For this review, take the finished solid that the model builds, in its own axes (mm). Give positions to 0.01 mm unless a question says otherwise; leave off trailing zeros. Loops run counter-clockwise (first coordinate to the right, second up) from the corner with the lowest first, then second, coordinate; pieces in that order, holes last. Notation, with made-up numbers: (35, 71) - (48, 71) arc R5 ccw to (48, 79) - close; hole circle Ø4 at (14.5, 80.5). An arc over 180 degrees is marked (long way). Answer in a Markdown table with one row per item.
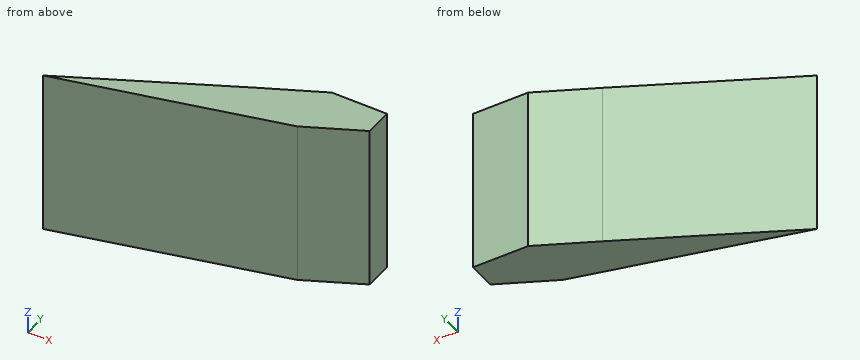
Autodesk Fusion 360 part; units mm, degrees
sketch "Sketch4" plane through (0, 0, 0) normal (0, 0, 1) x (1, 0, 0)
  line L0 (0, 0) -> (30, 0)
  line L1 (30, 0) -> (30, 10)
  line L2 (30, 10) -> (0, 10)
  line L3 (0, 10) -> (0, 0)
sketch "Sketch5" plane through (0, 0, 0) normal (0, 0, 1) x (1, 0, 0)
  line L0 (0, 0) -> (20, 5)
  line L1 (20, 5) -> (25.0128, 7.4566)
  line L2 (25.0128, 7.4566) -> (25.0128, 10)
  line L3 (25.0128, 10) -> (20, 10)
  line L4 (20, 10) -> (14.8103, 7.4566)
  line L5 (14.8103, 7.4566) -> (0, 0)
extrude "Extrude9" add sketch "Sketch5" along normal blind 15
1. We need section C-C, the plane y = 4. Give the boundary of the cut face in (x, z), and give its area (3 significant figures).
Values:
| item | result |
|---|---|
| outline | (7.94, 0) - (16, 0) - (16, 15) - (7.94, 15) - close |
| area | 121 mm^2 |
2. We need section B-B, the plane x = 2. Give the boundary of the cut face in (y, z), and give its area (3 significant figures).
Values:
| item | result |
|---|---|
| outline | (0.5, 0) - (1.01, 0) - (1.01, 15) - (0.5, 15) - close |
| area | 7.60 mm^2 |
3. Wall thickness on line 1 (Y direction, x = 17.25, z = 11.5); line 2 (Y direction, x = 1.75, z = 6.5); line 3 (X direction, y = 9.25, z = 13.5): over which ranges is each line inside the solid? List them lowest first. Write a range as [from, to].
Values:
| item | result |
|---|---|
| line 1 | y = [4.31, 8.65] |
| line 2 | y = [0.44, 0.88] |
| line 3 | x = [18.47, 25.01] |
4. We need section A-A, the plane z = 11.5. Give the boundary of the cut face in (x, y), and give its area (3 significant figures).
Values:
| item | result |
|---|---|
| outline | (0, 0) - (20, 5) - (25.01, 7.46) - (25.01, 10) - (20, 10) - (14.81, 7.46) - close |
| area | 69.4 mm^2 |
5. Clearance check with flat-ended pins moving along their axes: pin 1 (3 mm diameter, centred on x = 5.5, z = 4, fed in from +Y); pin 2 (1 mm diameter, centred on x = 19, z = 3.5, fed in from +Y). State where each tip first meets the part, or that it passes through.
Values:
| item | result |
|---|---|
| pin 1 | stops at y = 3.52 |
| pin 2 | stops at y = 9.75 |
